Input: dimensioned drawing with shaded views. Units: mm. Origin: part minimum x, y, z. A direction names the side the tool comes from. Give positions to 0.01 mm unless a question says otherwise; leave off trailing zeros. Write each loop counter-clockwise with the first axis right and the second up, starting at its lowest first coordinate (ties: lowest second). Pieces come first, ordered by that corner, then holes. Notation, with made-up numbers: (86.25, 71.25) -> (116.25, 71.25) arc R15 ccw to (116.25, 94.25) -> close; hole circle Ø6 at (13.5, -7). An arc over 180 degrees is marked (long way). Answer in a Markdown table with one row per item. Add a question column.
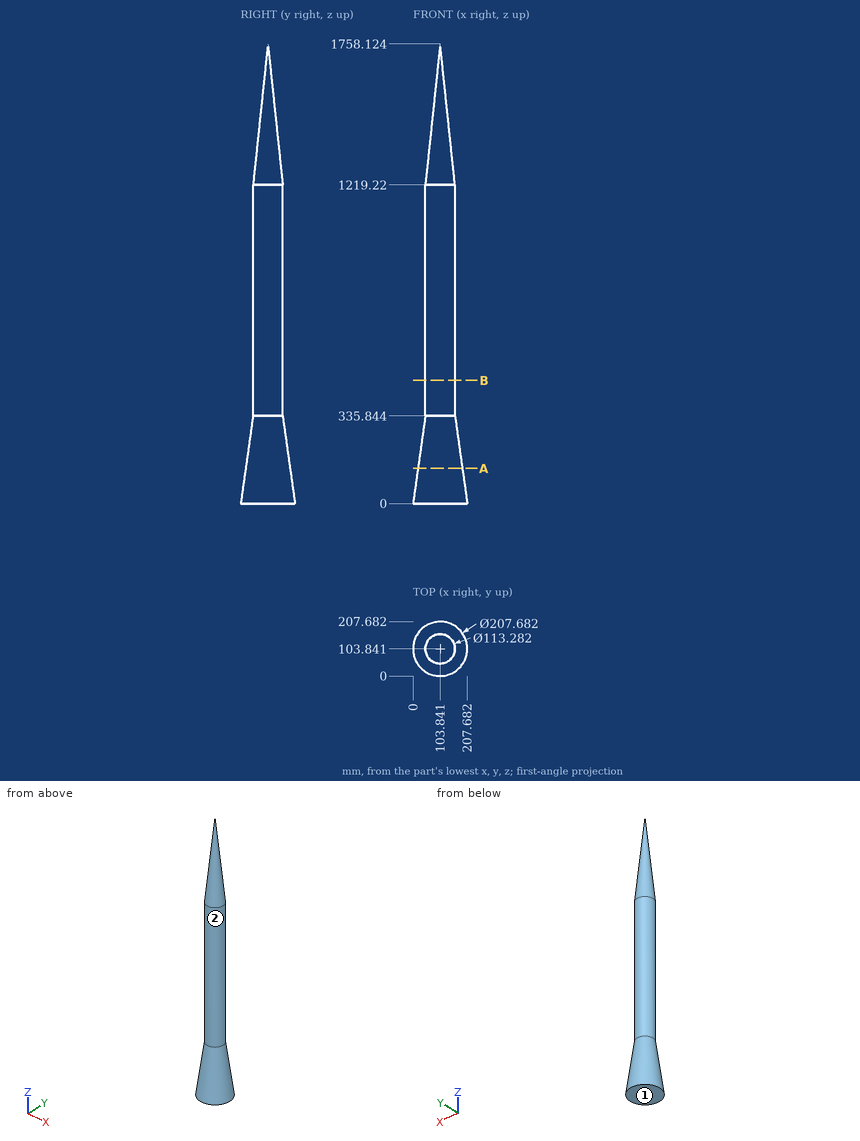
Q1. Contact query for flat-ended pins moving along their axis: pin 1 Ø12 at (y, z) = (76, 390.5) entering from +X; pin 2 Ø1.5 at (y, z) = (51.5, 748) entering from +X; pin 3 Ø8 at (y, z) = (115, 499.5) entering from -X; pin 4 Ø10 at (x, z) = (168.5, 1012.5) entering from +Y. Output: stop coordinate, or through.
Q2. Section A-A on z = 135.5. Return loops of the section in (x, y) (1 decimal).
Q3. Access query for the marked faces 1 and 2. Directions: +Z, -Z, +X, -X, +Y, -Y. A direction counts if a zero-diameter tool reaches every point of the face in a straight line with its end or side. Return the directions, or none.
Q4. Section B-B on z = 472. Return loops of the section in (x, y), and give its area (3 significant figures).
Q5. Line query: probe 1 along Y at (x, z) = (104, 926); probe 2 along Y at (x, z) = (139, 265); probe 3 along X at (y, z) = (114.5, 1398). Output: solid intervals per line, ascending. Write a range as from..to.
Checks:
| question | item | result |
|---|---|---|
| 1 | pin 1 | x = 156.1 |
| 1 | pin 2 | x = 127.22 |
| 1 | pin 3 | x = 47.65 |
| 1 | pin 4 | through |
| 2 | outline | circle Ø169.6 at (103.8, 103.8) |
| 3 | face 1 | -Z, +X, -X, +Y, -Y |
| 3 | face 2 | +Z |
| 4 | outline | circle Ø113.28 at (103.84, 103.84) |
| 4 | area | 10,100 mm^2 |
| 5 | probe 1 | 47.2..160.48 |
| 5 | probe 2 | 47.28..160.4 |
| 5 | probe 3 | 67.52..140.16 |
